The listing builds one solid part. Answer for the finished solid, in the listing's coordinates (mm). A direction names the side the tool comes from. Give positions to 0.01 mm unless a question says otherwise; leave off trailing zeros. Write each loop counter-clockwise with the first axis right and the second up, starting at its lowest first coordinate (ties: lowest second). Pieces come first, ordered by that corner, then holes. Notation, with made-up numbers: (4, 73.5) - (53, 73.5) arc R21 cw to (53, 97.5) - close; hole circle Ø5 at (-40, -17.5). An arc over 180 degrees is marked (long way). Return JSON: item names as keys, results as strings.
from build123d import *

# Parameters (mm, degrees)
SKETCH1_W           = 25
SKETCH1_H           = 62
SKETCH1_W_2         = 55
BOSS_EXTRUDE1_DEPTH = 4
SKETCH2_R           = 1.25
CUT_EXTRUDE1_DEPTH  = 4
BOSS_EXTRUDE2_START = 2
SKETCH3_R           = 3
SKETCH3_R_2         = 1.25
BOSS_EXTRUDE2_DEPTH = 2
SKETCH4_R           = 1.25
CUT_EXTRUDE2_DEPTH  = 10
BOSS_EXTRUDE3_START = 2
SKETCH5_R           = 3
SKETCH5_R_2         = 1.25
BOSS_EXTRUDE3_DEPTH = 2
LPATTERN1_COUNT     = 2
LPATTERN1_PITCH     = 25
SKETCH6_R           = 1.25
CUT_EXTRUDE3_DEPTH  = 75.520131508
BOSS_EXTRUDE4_START = 2
SKETCH7_R           = 3
SKETCH7_R_2         = 1.25
BOSS_EXTRUDE4_DEPTH = 2
SKETCH8_W           = 12.5
SKETCH8_H           = 12.5
CUT_EXTRUDE4_DEPTH  = 75.520131508
FILLET1_R           = 3
BOSS_EXTRUDE5_DEPTH = 2
SKETCH10_W          = 80
SKETCH10_H          = 9
BOSS_EXTRUDE6_DEPTH = 7
CHAMFER1_SIZE       = 2
SKETCH11_R          = 1.45
CUT_EXTRUDE5_DEPTH  = 7


with BuildPart() as part:
    # Sketch1 → Boss-Extrude1 (new body)
    with BuildSketch(Plane.XY):
        Rectangle(SKETCH1_W, SKETCH1_H)
        with Locations((40, 0)):
            Rectangle(SKETCH1_W_2, SKETCH1_H)
    extrude(amount=BOSS_EXTRUDE1_DEPTH)

    # Sketch2 → Cut-Extrude1 (cut)
    with BuildSketch(Plane.XY.offset(4)):
        with Locations((-9.5, -28)):
            Circle(SKETCH2_R)
        with Locations(Location((9.5, -28, 0), (0, 0, 180))):
            Circle(SKETCH2_R)
        with Locations((9.5, 28)):
            Circle(SKETCH2_R)
        with Locations(Location((-9.5, 28, 0), (0, 0, 180))):
            Circle(SKETCH2_R)
    extrude(amount=-CUT_EXTRUDE1_DEPTH, mode=Mode.SUBTRACT)

    # Sketch3 → Boss-Extrude2 (add)
    # profile 1 of 4: a face of its own
    with BuildSketch(Plane.XY.offset(4).offset(BOSS_EXTRUDE2_START)):
        with Locations(Location((-9.5, 28, 0), (0, 0, 180))):
            Circle(SKETCH3_R)
        with Locations((-9.5, 28)):
            Circle(SKETCH3_R_2, mode=Mode.SUBTRACT)
    # profile 2 of 4: a face of its own
    with BuildSketch(Plane.XY.offset(4).offset(BOSS_EXTRUDE2_START)):
        with Locations(Location((9.5, 28, 0), (0, 0, 90))):
            Circle(SKETCH3_R)
        with Locations((9.5, 28)):
            Circle(SKETCH3_R_2, mode=Mode.SUBTRACT)
    # profile 3 of 4: a face of its own
    with BuildSketch(Plane.XY.offset(4).offset(BOSS_EXTRUDE2_START)):
        with Locations(Location((-9.5, -28, 0), (0, 0, 180))):
            Circle(SKETCH3_R)
        with Locations((-9.5, -28)):
            Circle(SKETCH3_R_2, mode=Mode.SUBTRACT)
    # profile 4 of 4: a face of its own
    with BuildSketch(Plane.XY.offset(4).offset(BOSS_EXTRUDE2_START)):
        with Locations(Location((9.5, -28, 0), (0, 0, 270))):
            Circle(SKETCH3_R)
        with Locations((9.5, -28)):
            Circle(SKETCH3_R_2, mode=Mode.SUBTRACT)
    extrude(amount=-BOSS_EXTRUDE2_DEPTH)

    # Sketch4 → Cut-Extrude2 (cut)
    with BuildSketch(Plane.XY.offset(4)):
        with Locations((34.5, -12)):
            Circle(SKETCH4_R)
        with Locations((64.5, -28)):
            Circle(SKETCH4_R)
    cut_extrude2 = extrude(amount=-CUT_EXTRUDE2_DEPTH, mode=Mode.SUBTRACT)

    # Sketch5 → Boss-Extrude3 (add)
    # profile 1 of 2: a face of its own
    with BuildSketch(Plane.XY.offset(4).offset(BOSS_EXTRUDE3_START)):
        with Locations((34.5, -12)):
            Circle(SKETCH5_R)
        with Locations((34.5, -12)):
            Circle(SKETCH5_R_2, mode=Mode.SUBTRACT)
    # profile 2 of 2: a face of its own
    with BuildSketch(Plane.XY.offset(4).offset(BOSS_EXTRUDE3_START)):
        with Locations((64.5, -28)):
            Circle(SKETCH5_R)
        with Locations((64.5, -28)):
            Circle(SKETCH5_R_2, mode=Mode.SUBTRACT)
    boss_extrude3 = extrude(amount=-BOSS_EXTRUDE3_DEPTH)

    # LPattern1: Cut-Extrude2, Boss-Extrude3 ×2
    with Locations(*[(0, i * LPATTERN1_PITCH, 0) for i in range(1, LPATTERN1_COUNT)]):
        add(cut_extrude2, mode=Mode.SUBTRACT)
        add(boss_extrude3)

    # Sketch6 → Cut-Extrude3 (cut, through all)
    with BuildSketch(Plane(origin=(0, 0, 0), x_dir=(-1, 0, 0), z_dir=(0, 0, -1))):
        with Locations((-64.5, -12)):
            Circle(SKETCH6_R)
        with Locations((-34.5, -28)):
            Circle(SKETCH6_R)
        with Locations((-64.5, 13)):
            Circle(SKETCH6_R)
        with Locations((-34.5, -3)):
            Circle(SKETCH6_R)
    extrude(amount=-CUT_EXTRUDE3_DEPTH, mode=Mode.SUBTRACT)

    # Sketch7 → Boss-Extrude4 (add)
    # profile 1 of 4: a face of its own
    with BuildSketch(Plane(origin=(0, 0, 0), x_dir=(-1, 0, 0), z_dir=(0, 0, -1)).offset(BOSS_EXTRUDE4_START)):
        with Locations(Location((-64.5, 13, 0), (0, 0, 180))):
            Circle(SKETCH7_R)
        with Locations((-64.5, 13)):
            Circle(SKETCH7_R_2, mode=Mode.SUBTRACT)
    # profile 2 of 4: a face of its own
    with BuildSketch(Plane(origin=(0, 0, 0), x_dir=(-1, 0, 0), z_dir=(0, 0, -1)).offset(BOSS_EXTRUDE4_START)):
        with Locations(Location((-34.5, -3, 0), (0, 0, 180))):
            Circle(SKETCH7_R)
        with Locations((-34.5, -3)):
            Circle(SKETCH7_R_2, mode=Mode.SUBTRACT)
    # profile 3 of 4: a face of its own
    with BuildSketch(Plane(origin=(0, 0, 0), x_dir=(-1, 0, 0), z_dir=(0, 0, -1)).offset(BOSS_EXTRUDE4_START)):
        with Locations(Location((-34.5, -28, 0), (0, 0, 270))):
            Circle(SKETCH7_R)
        with Locations((-34.5, -28)):
            Circle(SKETCH7_R_2, mode=Mode.SUBTRACT)
    # profile 4 of 4: a face of its own
    with BuildSketch(Plane(origin=(0, 0, 0), x_dir=(-1, 0, 0), z_dir=(0, 0, -1)).offset(BOSS_EXTRUDE4_START)):
        with Locations(Location((-64.5, -12, 0), (0, 0, 180))):
            Circle(SKETCH7_R)
        with Locations((-64.5, -12)):
            Circle(SKETCH7_R_2, mode=Mode.SUBTRACT)
    extrude(amount=-BOSS_EXTRUDE4_DEPTH)

    # Sketch8 → Cut-Extrude4 (cut, through all)
    with BuildSketch(Plane.XY.offset(4)):
        with BuildLine():
            Line((5, 26), (-6.035898385, 26))
            ThreePointArc((-6.035898385, 26), (-6.671572875, 25.171572875), (-7.5, 24.535898385))
            Line((-7.5, 24.535898385), (-7.5, 13.5))
            Line((-7.5, 13.5), (5, 13.5))
            Line((5, 13.5), (5, 26))
        make_face()
        with BuildLine():
            ThreePointArc((12.964101615, 26), (11.920551066, 24.815516912), (10.5, 24.127016654))
            Line((10.5, 24.127016654), (10.5, 13.5))
            Line((10.5, 13.5), (23, 13.5))
            Line((23, 13.5), (23, 26))
            Line((23, 26), (12.964101615, 26))
        make_face()
        with BuildLine():
            Line((41, 26), (28.5, 26))
            Line((28.5, 26), (28.5, 13.5))
            Line((28.5, 13.5), (30.531373033, 13.5))
            ThreePointArc((30.531373033, 13.5), (34.5, 17), (38.468626967, 13.5))
            Line((38.468626967, 13.5), (41, 13.5))
            Line((41, 13.5), (41, 26))
        make_face()
        with Locations((52.75, 19.75)):
            Rectangle(SKETCH8_W, SKETCH8_H)
        with Locations((16.75, 1.75)):
            Rectangle(SKETCH8_W, SKETCH8_H)
        with BuildLine():
            Line((41, 8), (28.5, 8))
            Line((28.5, 8), (28.5, -4.5))
            Line((28.5, -4.5), (30.791900756, -4.5))
            ThreePointArc((30.791900756, -4.5), (34.5, 1), (38.208099244, -4.5))
            Line((38.208099244, -4.5), (41, -4.5))
            Line((41, -4.5), (41, 8))
        make_face()
        with Locations((52.75, 1.75)):
            Rectangle(SKETCH8_W, SKETCH8_H)
        with Locations((16.75, -16.25)):
            Rectangle(SKETCH8_W, SKETCH8_H)
        with BuildLine():
            Line((31.035898385, -10), (28.5, -10))
            Line((28.5, -10), (28.5, -22.5))
            Line((28.5, -22.5), (41, -22.5))
            Line((41, -22.5), (41, -10))
            Line((41, -10), (37.964101615, -10))
            ThreePointArc((37.964101615, -10), (34.5, -16), (31.035898385, -10))
        make_face()
        with Locations((52.75, -16.25)):
            Rectangle(SKETCH8_W, SKETCH8_H)
        with Locations((-1.25, 1.75)):
            Rectangle(SKETCH8_W, SKETCH8_H)
        with Locations((-1.25, -16.25)):
            Rectangle(SKETCH8_W, SKETCH8_H)
    extrude(amount=-CUT_EXTRUDE4_DEPTH, mode=Mode.SUBTRACT)

    # Fillet1
    fillet1_edges = [part.edges().sort_by_distance(p)[0] for p in [
        (67.5, 31, 2),
        (-12.5, 31, 2),
    ]]
    fillet(fillet1_edges, radius=FILLET1_R)

    # Sketch9 → Boss-Extrude5 (add)
    with BuildSketch(Plane.XZ.offset(31)):
        Polygon((-12.5, 0), (34.5, 0), (67.5, 0), (67.5, 4), (64.5, 4), (9.5, 4), (-9.5, 4), (-12.5, 4), align=None)
    extrude(amount=BOSS_EXTRUDE5_DEPTH)

    # Sketch10 → Boss-Extrude6 (add)
    with BuildSketch(Plane.XZ.offset(33)):
        with Locations((27.5, 2)):
            Rectangle(SKETCH10_W, SKETCH10_H)
    extrude(amount=BOSS_EXTRUDE6_DEPTH)

    # Chamfer1
    chamfer1_edges = [part.edges().sort_by_distance(p)[0] for p in [
        (27.5, -33, -2.5),
        (27.5, -33, 6.5),
    ]]
    chamfer(chamfer1_edges, length=CHAMFER1_SIZE)

    # Sketch11 → Cut-Extrude5 (cut)
    with BuildSketch(Plane.XZ.offset(40)):
        with Locations(Location((60, 2, 0), (0, 0, 270))):
            Circle(SKETCH11_R)
        with Locations(Location((-5, 2, 0), (0, 0, 90))):
            Circle(SKETCH11_R)
    extrude(amount=-CUT_EXTRUDE5_DEPTH, mode=Mode.SUBTRACT)


solid = part.part
Item 1: A cutting plane is placed at B-B on x = 27.5. Determine the outline of the cut face in (y, z).
Answer below:
{"outline": "(-40, -2.5) - (-35, -2.5) - (-33, -0.5) - (-33, 0) - (31, 0) - (31, 4) - (-33, 4) - (-33, 4.5) - (-35, 6.5) - (-40, 6.5) - close"}
Item 2: The mould has two halves that part along Y. Classify faces 1 (the face through (-7.5, 19, 2)), 2 (the face through (-4.12, -36.55, 0.85)), 3 (the face through (60, -33, 2)): +Y half, -Y half, draft (parallel to the pull), parting line (faces both ways), or undercut.
Answer below:
{"face 1": "undercut", "face 2": "draft", "face 3": "-Y half"}
Item 3: A cutting plane is placed at A-A on x = 55. Determine the outline of the cut face in (y, z).
Answer below:
{"outline": "(-40, -2.5) - (-35, -2.5) - (-33, -0.5) - (-33, 0) - (-22.5, 0) - (-22.5, 4) - (-33, 4) - (-33, 4.5) - (-35, 6.5) - (-40, 6.5) - close; (-10, 0) - (-4.5, 0) - (-4.5, 4) - (-10, 4) - close; (8, 0) - (13.5, 0) - (13.5, 4) - (8, 4) - close; (26, 0) - (31, 0) - (31, 4) - (26, 4) - close"}
Item 4: A cutting plane is placed at C-C on z = 2. Give the number of separate pieces and of enclosed holes in the cut face, then the cut area to 3 significant figures.
Answer below:
{"separate pieces": "1", "enclosed holes": "24", "area": "3,800 mm²"}
Item 5: For faces 4 (the face through (53, 8, 2)), 5 (the face through (66, -3, 6)), 6 (the face through (61.5, 12.9, -1)), determine the directions among +Z, -Z, +X, -X, +Y, -Y from which every point of the face is accessible in a straight line to the end or side of a thin tool.
Answer below:
{"face 4": "+Z, -Z", "face 5": "+Z, +X, -X, +Y", "face 6": "-Z"}
Item 6: Consider L1, parallel to Y at x = 1.5, z = 3; L2, parallel to Z at x = -5, y = -35.75; L3, parallel to Y at x = 10.5, z = 5.25. Determine where each line is inside the solid, lowest interval first.
Answer below:
{"L1": "y = -40 to -22.5, -10 to -4.5, 8 to 13.5, 26 to 31", "L2": "z = -2.5 to 0.55, 3.45 to 6.5", "L3": "y = -40 to -33.75, -30.83 to -28.75, -27.25 to -25.17, 25.17 to 27.25, 28.75 to 30.83"}
Item 7: Flat-ended cylindrical pins translate along their axes: P1, Ø3, axis at x = -4.5, z = 2.5, coming from the -Y side; P2, Ø3, axis at x = 64.5, y = 14, coming from the -Z side; P3, Ø5, axis at x = 63.5, y = -28, coming from the +Z side; P4, Ø12, axis at x = 54.5, y = -20, coming from the -Z side. Find the tip coordinate at first contact, or state that the pin passes through.
Answer below:
{"P1": "stops at y = -40", "P2": "stops at z = -2", "P3": "stops at z = 6", "P4": "stops at z = 0"}
